from build123d import *

# Parameters (mm, degrees)
RESSALTO_EXTRUS_O1_DEPTH = 3


with BuildPart() as part:
    # Esboço1 → Ressalto-extrusão1 (new body)
    with BuildSketch(Plane.XY):
        with BuildLine():
            Line((19, 0), (12.625, 0))
            Line((12.625, 0), (12.625, 5.15))
            Line((12.625, 5.15), (11, 5.15))
            Line((11, 5.15), (8, 5.15))
            Line((8, 5.15), (6.375, 5.15))
            Line((6.375, 5.15), (6.375, 0))
            Line((6.375, 0), (0, 0))
            Line((0, 0), (0.448555141, 6.151613366))
            ThreePointArc((0.448555141, 6.151613366), (0.584055906, 8.075483405), (0.710041083, 10))
            add(Edge.make_bspline(
                [(0.710041083, 10), (2.087312964, 19.459463986), (8, 20)],
                knots=[0, 0, 0, 0.891892797, 0.891892797, 0.891892797], degree=2))
            Line((8, 20), (8, 10))
            Line((8, 10), (11, 10))
            Line((11, 10), (11, 20))
            add(Edge.make_bspline(
                [(18.289958917, 10), (16.912687036, 19.459463986), (11, 20)],
                knots=[0, 0, 0, 0.891892797, 0.891892797, 0.891892797], degree=2))
            ThreePointArc((18.289958917, 10), (18.415944094, 8.075483405), (18.551444859, 6.151613366))
            Line((18.551444859, 6.151613366), (19, 0))
        make_face()
    extrude(amount=RESSALTO_EXTRUS_O1_DEPTH)


solid = part.part
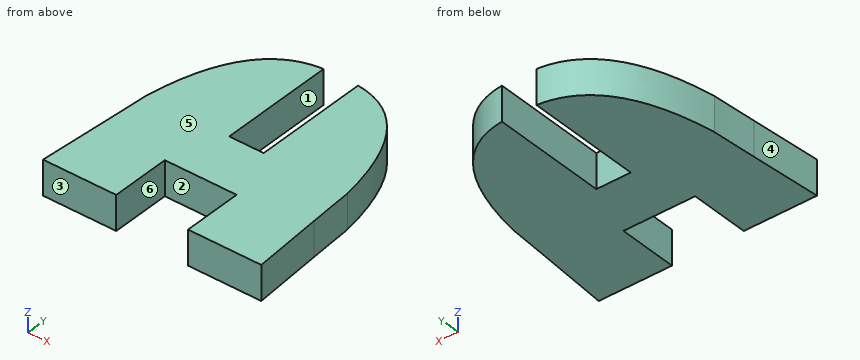
Verification items for the finished model (mm, model axes). Face numbers are marked on the shaded views. A direction names the side the tool comes from. Round coordinates to 2 decimals unless told otherwise and drop trailing zeros. Loops run counter-clockwise (first coordinate to the right, second up) from the corner with the lowest first, then second, coordinate; pieces in that order, holes last. Notation, with made-up numbers: M 12,-6.75 L 61,-6.75 A5 cw 61,-1.75 Z; hole C 7,-37.75 d4. An arc over 180 degrees is marked long. Write each question's results on one line, items separated by ' | '.
1) Mould release check, pull along X, two halves, no side actions. Record for the marked faces 4, 5 and 6: released by +X, released by -X, zero draft, split by the parting line, or undercut.
Checks:
face 4: released by -X | face 5: zero draft | face 6: undercut
2) Section check C-C on y = 7.75. Record the boundary of the cut face in (x, z), then the cut area to 3 significant figures.
Checks:
outline: M 0.56,0 L 18.44,0 L 18.44,3 L 0.56,3 Z | area: 53.6 mm2
3) Gauge pin test, flat ends, axial feed: P1, Ø0.9, axis at y = 2.5, z = 1, coming from the +X side; P2, Ø0.9, axis at y = 2.5, z = 2, coming from the -X side; P3, Ø1.5, axis at y = 15, z = 1, coming from the -X side. Record the tip position at first contact, or that the pin passes through.
Checks:
P1: stops at x = 18.85 | P2: stops at x = 0.15 | P3: stops at x = 1.71
4) Scan lines: L1, parallel to Y at x = 10.5, z = 2.1; L2, parallel to X at y = 3.75, z = 1.35 (3 decimals); L3, parallel to X at y = 2, z = 2.4 (3 decimals). Record each from-to range of solid material in increasing order. Write a range as from..to.
Checks:
L1: y = 5.15..10 | L2: x = 0.273..6.375, 12.625..18.727 | L3: x = 0.146..6.375, 12.625..18.854
5) Access from +Z, -Z, +X, -X, +Y, -Y to the whole of each face (thin tool, end or side, straight path). Record for the marked faces 1, 2 and 3.
Checks:
face 1: +Z, -Z, +Y | face 2: +Z, -Z, -Y | face 3: +Z, -Z, +X, -X, -Y
6) Section check B-B on x = 9.5. Record the boundary of the cut face in (y, z), then the cut area to 4 significant figures.
Checks:
outline: M 5.15,0 L 10,0 L 10,3 L 5.15,3 Z | area: 14.55 mm2
7) Section check A-A on y = 4.25. Record the boundary of the cut face in (x, z) (3 decimals).
Checks:
outline: M 0.31,0 L 6.375,0 L 6.375,3 L 0.31,3 Z; M 12.625,0 L 18.69,0 L 18.69,3 L 12.625,3 Z
